from build123d import *

# Parameters (mm, degrees)
BOSS_EXTRUDE1_START = -5
BOSS_EXTRUDE1_DEPTH = 10
SKETCH5_R           = 1.75
CUT_EXTRUDE1_DEPTH  = 10.848857802
SKETCH6_R           = 1.75
CUT_EXTRUDE2_DEPTH  = 10.848857802


with BuildPart() as part:
    # Sketch4 → Boss-Extrude1 (new body)
    with BuildSketch(Plane.XY.offset(BOSS_EXTRUDE1_START)):
        with BuildLine():
            Line((-6, 6), (-6, -6))
            Line((-6, -6), (6, -6))
            Line((6, -6), (6, -4.5))
            ThreePointArc((6, -4.5), (5.853553391, -4.146446609), (5.5, -4))
            Line((5.5, -4), (-3.5, -4))
            ThreePointArc((-3.5, -4), (-3.853553391, -3.853553391), (-4, -3.5))
            Line((-4, -3.5), (-4, 5.5))
            ThreePointArc((-4, 5.5), (-4.146446609, 5.853553391), (-4.5, 6))
            Line((-4.5, 6), (-6, 6))
        make_face()
    extrude(amount=BOSS_EXTRUDE1_DEPTH)

    # Sketch5 → Cut-Extrude1 (cut, through all)
    with BuildSketch(Plane(origin=(0, 0, 0), x_dir=(0, 0, -1), z_dir=(1, 0, 0))):
        Circle(SKETCH5_R)
    extrude(amount=-CUT_EXTRUDE1_DEPTH, mode=Mode.SUBTRACT)

    # Sketch6 → Cut-Extrude2 (cut, through all)
    with BuildSketch(Plane(origin=(0, 0, 0), x_dir=(1, 0, 0), z_dir=(0, 1, 0))):
        with Locations(Location((0, 0, 0), (0, 0, 270))):
            Circle(SKETCH6_R)
    extrude(amount=-CUT_EXTRUDE2_DEPTH, mode=Mode.SUBTRACT)


solid = part.part
Geometry: final body of the model. Coordinates: model frame, mm. A direction names the side the tool comes from. Give positions to 0.01 mm unless a question says otherwise; leave off trailing zeros. Write each loop counter-clockwise with the first axis right and the second up, starting at its lowest first coordinate (ties: lowest second). Pieces come first, ordered by that corner, then holes. Notation, with made-up numbers: M -27,75.25 L 32,75.25 A19 cw 32,93.25 Z; hole C 10,54 d2. An arc over 180 degrees is marked long. Answer in a Markdown table with one row per item. Add a question column.
(1) Ray query, line 1 (X direction, y = -5.3, z = 0); line 2 (X direction, y = -3.25, z = 0.5). Return the intervals inside material, ascending.
(2) Reachability of faces 1 (the flat face through (-4, 2, 0)), 2 (the cylindrical face through (-4.986, -0.67, -1.617)) from +Z, -Z, +X, -X, +Y, -Y: full face, straight path, thin tool, end or side. Return the list, or none.
(3) First-contact query: pin 1 (4.5 mm diameter, centred on y = 2.5, z = 1, fed in from +X); pin 2 (1.5 mm diameter, centred on x = 4, z = -1, fed in from +Y); pin 3 (2 mm diameter, centred on y = 0, z = 0, fed in from +X). Flat tips, straight axial feed; report the tip coordinate or a pass-through.
(4) Section C-C on z = 0. Return loops of the section in (x, y), and give its area (3 significant figures).
(5) Mould query, pull axis Z, two halves, no side actions, for faces 3 (the flat face through (-4.5, -2.2, -5)), 4 (the cylindrical face through (-1.71, -4.99, -0.38)), 5 (the flat face through (2, -4, 0)). Classes: +Z half, -Z half, draft (parallel to the pull), parting line (faces both ways), or undercut.
(6) Section D-D on z = 4. Return loops of the section in (x, y), and give its area (3 significant figures).
(7) Section A-A on x = 0. Return loops of the section in (y, z), and give its area (3 significant figures).
Result set:
| question | item | result |
|---|---|---|
| 1 | line 1 | x = -6 to -1.75, 1.75 to 6 |
| 1 | line 2 | x = -6 to -4 |
| 2 | face 1 | +Z, -Z, +X, +Y |
| 2 | face 2 | +X, -X |
| 3 | pin 1 | stops at x = -4 |
| 3 | pin 2 | stops at y = -4 |
| 3 | pin 3 | passes through |
| 4 | outline | M -6,-6 L -1.75,-6 L -1.75,-4 L -3.5,-4 A0.5 cw -4,-3.5 L -4,-1.75 L -6,-1.75 Z; M -6,1.75 L -4,1.75 L -4,5.5 A0.5 ccw -4.5,6 L -6,6 Z; M 1.75,-6 L 6,-6 L 6,-4.5 A0.5 ccw 5.5,-4 L 1.75,-4 Z |
| 4 | area | 29.9 mm^2 |
| 5 | face 3 | -Z half |
| 5 | face 4 | undercut |
| 5 | face 5 | draft |
| 6 | outline | M -6,-6 L 6,-6 L 6,-4.5 A0.5 ccw 5.5,-4 L -3.5,-4 A0.5 cw -4,-3.5 L -4,5.5 A0.5 ccw -4.5,6 L -6,6 Z |
| 6 | area | 43.9 mm^2 |
| 7 | outline | M -6,-5 L -4,-5 L -4,-1.75 L -6,-1.75 Z; M -6,1.75 L -4,1.75 L -4,5 L -6,5 Z |
| 7 | area | 13.0 mm^2 |
